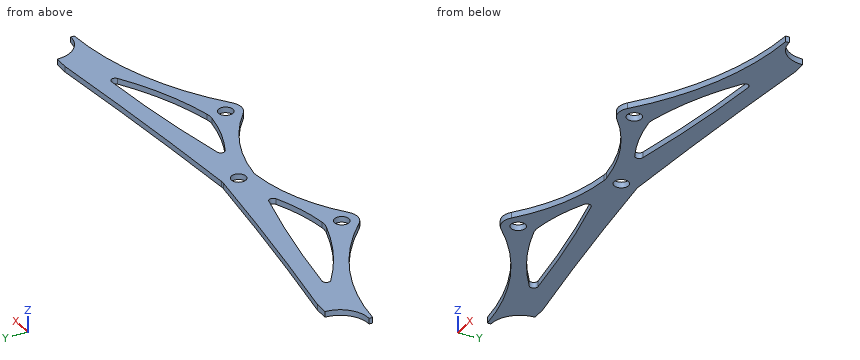
from build123d import *

# Parameters (mm, degrees)
PLANETARY_START           = -12.7
SKETCH1207_R              = 3.25
SKETCH1207_R_2            = 3.250000002
PLANETARY_INNER_TAB_DEPTH = 2.54
SMAL_ANGLE_FILLET_R       = 1.778
LARGE_ANGLE_FILLET_R      = 10.16


with BuildPart() as part:
    # Sketch1207 → Planetary Inner Tab (new body)
    with BuildSketch(Plane.XY.offset(PLANETARY_START)):
        with BuildLine():
            Line((-1653.472019465, 334.01), (-1653.472019465, 332.4225))
            ThreePointArc((-1653.472019465, 332.4225), (-1617.417278513, 323.366740441), (-1586.500499811, 302.724455656))
            ThreePointArc((-1586.500499811, 302.724455656), (-1581.895902138, 300.801653447), (-1577.180577212, 302.434197141))
            ThreePointArc((-1577.180577212, 302.434197141), (-1556.772529786, 314.866684199), (-1533.595059081, 320.685617601))
            ThreePointArc((-1533.595059081, 320.685617601), (-1510.41725967, 314.866679973), (-1490.008857704, 302.434160123))
            ThreePointArc((-1490.008857704, 302.434160123), (-1485.502791315, 300.798266511), (-1481.000799136, 302.445339259))
            ThreePointArc((-1481.000799136, 302.445339259), (-1446.058878011, 323.434373498), (-1406.300973236, 332.4225))
            Line((-1406.300973236, 332.4225), (-1406.300973236, 334.01))
            ThreePointArc((-1406.300973236, 334.01), (-1415.281229357, 337.729743879), (-1419.000973236, 346.71))
            Line((-1419.000973236, 346.71), (-1425.350973236, 346.71))
            ThreePointArc((-1425.350973236, 346.71), (-1479.405888247, 340.173785728), (-1533.583149601, 334.74421061))
            ThreePointArc((-1533.583149601, 334.744210609), (-1584.077440056, 340.096278026), (-1634.422019465, 346.71))
            Line((-1634.422019465, 346.71), (-1640.772019465, 346.71))
            ThreePointArc((-1640.772019465, 346.71), (-1644.491763344, 337.729743879), (-1653.472019465, 334.01))
        make_face()
        with Locations((-1581.678000655, 307.798261121)):
            Circle(SKETCH1207_R, mode=Mode.SUBTRACT)
        with Locations((-1485.511478414, 307.798261121)):
            Circle(SKETCH1207_R, mode=Mode.SUBTRACT)
        with BuildLine():
            ThreePointArc((-1581.138275137, 314.881124344), (-1604.565453937, 323.676576229), (-1625.585402649, 337.254294614))
            ThreePointArc((-1625.585402649, 337.254294614), (-1587.708607657, 332.221823862), (-1550.251821341, 324.674207047))
            ThreePointArc((-1550.251821341, 324.674207047), (-1565.191775687, 318.190391811), (-1581.138275137, 314.881124344))
        make_face(mode=Mode.SUBTRACT)
        with Locations((-1533.595063997, 327.714985503)):
            Circle(SKETCH1207_R_2, mode=Mode.SUBTRACT)
        with BuildLine():
            ThreePointArc((-1516.716796741, 324.550332905), (-1477.373328625, 332.055126671), (-1437.619544261, 336.940517311))
            ThreePointArc((-1437.619544261, 336.940517311), (-1460.647521819, 323.41294144), (-1485.95203842, 314.871015491))
            ThreePointArc((-1485.95203842, 314.871015491), (-1501.829474856, 318.137183344), (-1516.716796741, 324.550332905))
        make_face(mode=Mode.SUBTRACT)
    extrude(amount=-PLANETARY_INNER_TAB_DEPTH)

    # Smal Angle Fillet
    smal_angle_fillet_edges = [part.edges().sort_by_distance(p)[0] for p in [
        (-1550.251821341, 324.674207047, -13.97),
        (-1625.585402649, 337.254294614, -13.97),
        (-1437.619544261, 336.940517311, -13.97),
        (-1516.716796741, 324.550332905, -13.97),
    ]]
    fillet(smal_angle_fillet_edges, radius=SMAL_ANGLE_FILLET_R)

    # Large Angle Fillet
    large_angle_fillet_edges = [part.edges().sort_by_distance(p)[0] for p in [
        (-1581.138275137, 314.881124344, -13.97),
        (-1533.595059081, 320.685617601, -13.97),
        (-1533.583149601, 334.744210609, -13.97),
        (-1485.95203842, 314.871015491, -13.97),
    ]]
    fillet(large_angle_fillet_edges, radius=LARGE_ANGLE_FILLET_R)


solid = part.part
Verification items for the finished model (mm, model axes). Round coordinates to 2 decimals unless told otherwise and drop trailing zeros. Loops run counter-clockwise (first coordinate to the right, second up) from the corner with the lowest first, then second, coordinate; pieces in that order, holes last. Notation, with made-up numbers: (13, 88) - (72, 88) arc R18 cw to (72, 92) - close; hole circle Ø11 at (2.25, 33). An arc over 180 degrees is marked (long way). Use a Markdown table: item, result. Add a question column.
1. Section check D-D, the plane z = -13.25. Give the number of separate pieces and of enclosed holes in the cut face, plus the area to 3 significant figures.
2. Thickness scan on probe 1 along X at (y, z) = (321, -13.45); probe 2 along X at (y, z) = (310.5, -13.55); probe 3 along X at (y, z) = (323, -14.2). Record the ranges inside material, lowest first. Write a range as [from, to].
3. Gauge pin test, flat end, axial feed: pin 1 (8 mm diameter, centred on x = -1523.5, y = 339.5, fed in from -Z). Record the tip position at first contact, or that the pin passes through.
4. Section check A-A, the plane y = 339.5. Record the boundary of the cut face in (x, z), plus the area to 3 significant figures.
5. Section check B-B, the plane x = -1498.5. Record the boundary of the cut face in (y, z).
6. Section check C-C, the plane y = 318.5. Record the boundary of the cut face in (x, z).
Checks:
| question | item | result |
|---|---|---|
| 1 | separate pieces | 1 |
| 1 | enclosed holes | 5 |
| 1 | area | 3,960 mm^2 |
| 2 | probe 1 | x = [-1612.43, -1598.87], [-1557.67, -1509.52], [-1466.28, -1451.73] |
| 2 | probe 2 | x = [-1595.64, -1583.48], [-1579.87, -1565.62], [-1501.57, -1487.32], [-1483.71, -1470.37] |
| 2 | probe 3 | x = [-1616.6, -1603.2], [-1553.88, -1513.09], [-1461.56, -1447.13] |
| 3 | pin 1 | stops at z = -15.24 |
| 4 | outline | (-1643.02, -15.24) - (-1579, -15.24) - (-1579, -12.7) - (-1643.02, -12.7) - close; (-1485.57, -15.24) - (-1416.76, -15.24) - (-1416.76, -12.7) - (-1485.57, -12.7) - close |
| 4 | area | 337 mm^2 |
| 5 | outline | (308.65, -15.24) - (317.17, -15.24) - (317.17, -12.7) - (308.65, -12.7) - close; (328.36, -15.24) - (338.13, -15.24) - (338.13, -12.7) - (328.36, -12.7) - close |
| 6 | outline | (-1607.76, -15.24) - (-1592.68, -15.24) - (-1592.68, -12.7) - (-1607.76, -12.7) - close; (-1564.24, -15.24) - (-1545.99, -15.24) - (-1545.99, -12.7) - (-1564.24, -12.7) - close; (-1521.2, -15.24) - (-1502.95, -15.24) - (-1502.95, -12.7) - (-1521.2, -12.7) - close; (-1473.05, -15.24) - (-1456.88, -15.24) - (-1456.88, -12.7) - (-1473.05, -12.7) - close |
